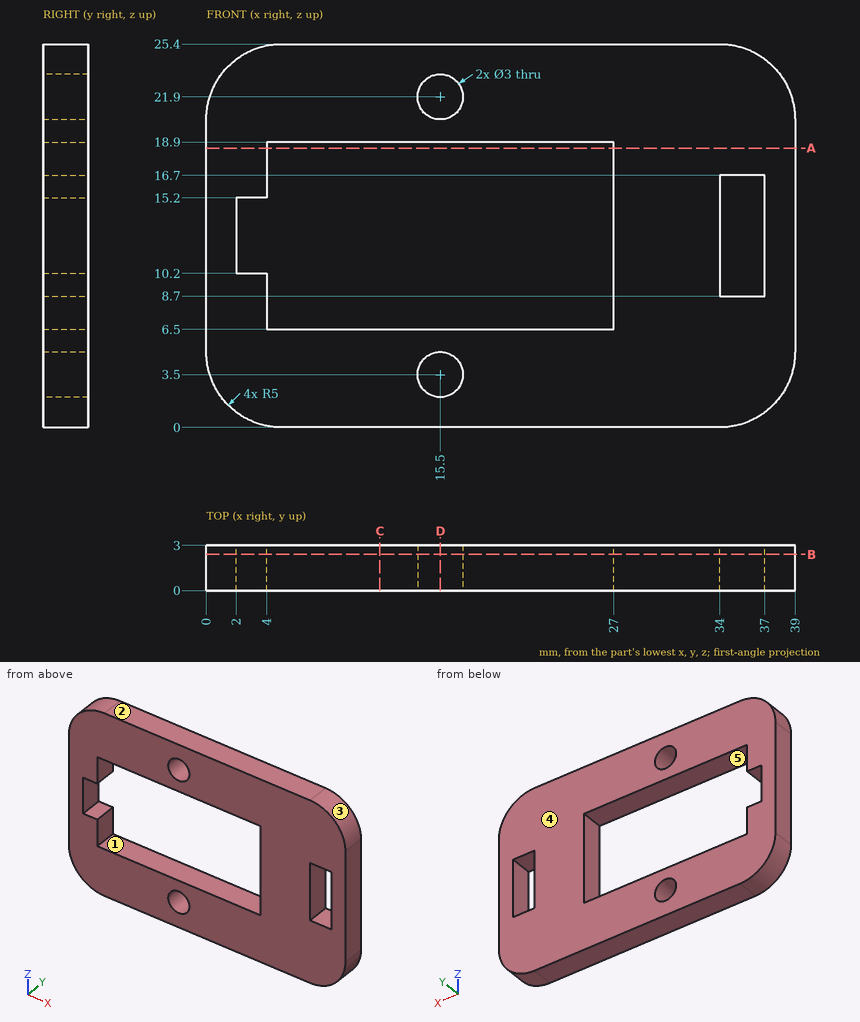
Source: three-view drawing plus pictorial views. Frame: mm from the lowest corner of the part. A direction names the side the tool comes from. Round coordinates to 2 decimals unless told otherwise and drop trailing zeros. Loops run counter-clockwise (first coordinate to the right, second up) from the corner with the lowest first, then second, coordinate; pieces in that order, holes last.
1. Access query for the marked faces 4 and 5. Directions: +Z, -Z, +X, -X, +Y, -Y. A direction counts if a zero-diameter tool reaches every point of the face in a straight line with its end or side. Return the directions, or none.
2. Mould query, pull axis X, two halves, no side actions, for the marked faces 1, 2 and 3. Classes: released by +X, released by -X, zero draft, split by the parting line, or undercut.
3. Section query A-A on z = 18.5. Output: boundary loops of the cut face in (x, y).
4. Contact query for flat-ended pins moving along their axis: pin 1 (1 mm diameter, centred on x = 3, y = 1.5, fed in from -Z); pin 2 (1.6 mm diameter, centred on x = 3, y = 1.5, fed in from +Z); pin 3 (1.5 mm diameter, centred on x = 35.5, y = 1.5, fed in from -Z). Output: stop coordinate, or through.
5. Ray query, L1, parallel to X at y = 1.35, z = 15.25; L2, parallel to X at y = 2.15, z = 11; L3, parallel to X at y = 2.65, z = 7.25. Return the intervals inside material, ascending.
6. Section query B-B on y = 2.4. Output: boundary loops of the cut face in (x, z).
7. Section query C-C on x = 11.5. Output: boundary loops of the cut face in (y, z).
8. Section query D-D on x = 15.5. Output: boundary loops of the cut face in (y, z), and give its area (3 significant figures).
Answers below:
1. face 4: +Z, -Z, +X, -X, +Y
1. face 5: +Y, -Y
2. face 1: undercut
2. face 2: zero draft
2. face 3: released by +X
3. outline: (0, 0) - (4, 0) - (4, 3) - (0, 3) - close; (27, 0) - (39, 0) - (39, 3) - (27, 3) - close
4. pin 1: stops at z = 0.23
4. pin 2: stops at z = 25.25
4. pin 3: stops at z = 0.06
5. L1: x = 0 to 4, 27 to 34, 37 to 39
5. L2: x = 0 to 2, 27 to 34, 37 to 39
5. L3: x = 0 to 4, 27 to 39
6. outline: (0, 5) arc R5 ccw to (5, 0) - (34, 0) arc R5 ccw to (39, 5) - (39, 20.4) arc R5 ccw to (34, 25.4) - (5, 25.4) arc R5 ccw to (0, 20.4) - close; hole (2, 10.2) - (4, 10.2) - (4, 6.5) - (27, 6.5) - (27, 18.9) - (4, 18.9) - (4, 15.2) - (2, 15.2) - close; hole circle Ø3 at (15.5, 3.5); hole circle Ø3 at (15.5, 21.9); hole (34, 8.7) - (37, 8.7) - (37, 16.7) - (34, 16.7) - close
7. outline: (0, 0) - (3, 0) - (3, 6.5) - (0, 6.5) - close; (0, 18.9) - (3, 18.9) - (3, 25.4) - (0, 25.4) - close
8. outline: (0, 0) - (3, 0) - (3, 2) - (0, 2) - close; (0, 5) - (3, 5) - (3, 6.5) - (0, 6.5) - close; (0, 18.9) - (3, 18.9) - (3, 20.4) - (0, 20.4) - close; (0, 23.4) - (3, 23.4) - (3, 25.4) - (0, 25.4) - close
8. area: 21.0 mm2
